Could you check a few things on this model? Use its own coordinates, in mm. A direction names the side the tool comes from. Coordinates: 2 decimals unless noted, no trailing zeros. One line per question, with ' | ' between items. Start each with the question number.
(1) Which directions (+Z, -Z, +X, -X, +Y, -Y) give clear straight access to the entire face, cutting with the end or side of a thin tool? Please do faces 1 (the face through (-72.28, 1.01, -83.14)), 2 (the face through (72.28, 1.01, 83.14)), 3 (the face through (-58.285, 1.014, -97.427)), 4 (the face through (60.1, 1, 85.3)).
(2) Suppose I cut it at A-A (y = 1.15). Give the number of separate pieces and of enclosed holes in the cut face, plus the area to 3 significant figures.
(3) If I drill on line 1 along Z through (x, y) = (-22, 1.9); line 2 along X through (y, z) = (1.2, -13.5); line 3 along X through (y, z) = (0.2, 96), over which ranges is the centre line in solid material (lowest first)?
(4) If we mould it in two halves opening along X, with no side actions, what happens to faces 5 (the face through (-1, 0, -1)), 6 (the face through (72.28, 1.01, -83.14)), 7 (the face through (-58.285, 1.014, 97.427))? For each: pulls with the +X half, pulls with the -X half, needs draft (parallel to the pull), parting line crosses it, or undercut.
```python
from build123d import *

# Parameters (mm, degrees)
SKETCH2_W           = 160
SKETCH2_H           = 210
SKETCH2_R           = 1.3
BOSS_EXTRUDE1_DEPTH = 2
SKETCH3_W           = 14
SKETCH3_H           = 20
CUT_EXTRUDE1_DEPTH  = 2
FILLET1_R           = 1.5
SKETCH4_R           = 1.3
CUT_EXTRUDE2_DEPTH  = 2
CUT_EXTRUDE3_DEPTH  = 2
SKETCH6_R           = 1.65
CUT_EXTRUDE4_DEPTH  = 2


with BuildPart() as part:
    # Sketch2 → Boss-Extrude1 (new body)
    with BuildSketch(Plane(origin=(0, 0, 0), x_dir=(1, 0, 0), z_dir=(0, 1, 0))):
        Rectangle(SKETCH2_W, SKETCH2_H)
        with Locations(Location((52.422835534, 88.736544033, 0), (0, 0, 270))):
            Circle(SKETCH2_R, mode=Mode.SUBTRACT)
        with Locations(Location((52.422835534, 96.514718626, 0), (0, 0, 270))):
            Circle(SKETCH2_R, mode=Mode.SUBTRACT)
        with Locations(Location((58.079689783, 102.171572875, 0), (0, 0, 270))):
            Circle(SKETCH2_R, mode=Mode.SUBTRACT)
        with Locations(Location((76, 13.5, 0), (0, 0, 270))):
            Circle(SKETCH2_R, mode=Mode.SUBTRACT)
        with Locations(Location((68, 13.5, 0), (0, 0, 270))):
            Circle(SKETCH2_R, mode=Mode.SUBTRACT)
        with Locations(Location((62.5, 8, 0), (0, 0, 270))):
            Circle(SKETCH2_R, mode=Mode.SUBTRACT)
        with Locations(Location((62.5, -8, 0), (0, 0, 90))):
            Circle(SKETCH2_R, mode=Mode.SUBTRACT)
        with Locations(Location((68, -13.5, 0), (0, 0, 90))):
            Circle(SKETCH2_R, mode=Mode.SUBTRACT)
        with Locations(Location((76, -13.5, 0), (0, 0, 90))):
            Circle(SKETCH2_R, mode=Mode.SUBTRACT)
        with Locations(Location((77.171572875, 83.079689783, 0), (0, 0, 90))):
            Circle(SKETCH2_R, mode=Mode.SUBTRACT)
        with Locations(Location((71.514718626, 77.422835534, 0), (0, 0, 90))):
            Circle(SKETCH2_R, mode=Mode.SUBTRACT)
        with Locations(Location((63.736544033, 77.422835534, 0), (0, 0, 90))):
            Circle(SKETCH2_R, mode=Mode.SUBTRACT)
        with Locations(Location((77.171572875, -83.079689783, 0), (0, 0, 270))):
            Circle(SKETCH2_R, mode=Mode.SUBTRACT)
        with Locations(Location((71.514718626, -77.422835534, 0), (0, 0, 270))):
            Circle(SKETCH2_R, mode=Mode.SUBTRACT)
        with Locations(Location((63.736544033, -77.422835534, 0), (0, 0, 270))):
            Circle(SKETCH2_R, mode=Mode.SUBTRACT)
        with Locations(Location((58.079689783, -102.171572875, 0), (0, 0, 90))):
            Circle(SKETCH2_R, mode=Mode.SUBTRACT)
        with Locations(Location((52.422835534, -96.514718626, 0), (0, 0, 90))):
            Circle(SKETCH2_R, mode=Mode.SUBTRACT)
        with Locations(Location((52.422835534, -88.736544033, 0), (0, 0, 90))):
            Circle(SKETCH2_R, mode=Mode.SUBTRACT)
        with Locations(Location((-58.079689783, 102.171572875, 0), (0, 0, 90))):
            Circle(SKETCH2_R, mode=Mode.SUBTRACT)
        with Locations(Location((-52.422835534, 96.514718626, 0), (0, 0, 90))):
            Circle(SKETCH2_R, mode=Mode.SUBTRACT)
        with Locations(Location((-52.422835534, 88.736544033, 0), (0, 0, 90))):
            Circle(SKETCH2_R, mode=Mode.SUBTRACT)
        with Locations(Location((-77.171572875, 83.079689783, 0), (0, 0, 270))):
            Circle(SKETCH2_R, mode=Mode.SUBTRACT)
        with Locations(Location((-71.514718626, 77.422835534, 0), (0, 0, 270))):
            Circle(SKETCH2_R, mode=Mode.SUBTRACT)
        with Locations(Location((-63.736544033, 77.422835534, 0), (0, 0, 270))):
            Circle(SKETCH2_R, mode=Mode.SUBTRACT)
        with Locations(Location((-77.171572875, -83.079689783, 0), (0, 0, 90))):
            Circle(SKETCH2_R, mode=Mode.SUBTRACT)
        with Locations(Location((-71.514718626, -77.422835534, 0), (0, 0, 90))):
            Circle(SKETCH2_R, mode=Mode.SUBTRACT)
        with Locations(Location((-63.736544033, -77.422835534, 0), (0, 0, 90))):
            Circle(SKETCH2_R, mode=Mode.SUBTRACT)
        with Locations(Location((-52.422835534, -88.736544033, 0), (0, 0, 270))):
            Circle(SKETCH2_R, mode=Mode.SUBTRACT)
        with Locations(Location((-52.422835534, -96.514718626, 0), (0, 0, 270))):
            Circle(SKETCH2_R, mode=Mode.SUBTRACT)
        with Locations(Location((-58.079689783, -102.171572875, 0), (0, 0, 270))):
            Circle(SKETCH2_R, mode=Mode.SUBTRACT)
        with Locations(Location((-62.5, -8, 0), (0, 0, 270))):
            Circle(SKETCH2_R, mode=Mode.SUBTRACT)
        with Locations(Location((-68, -13.5, 0), (0, 0, 270))):
            Circle(SKETCH2_R, mode=Mode.SUBTRACT)
        with Locations(Location((-76, -13.5, 0), (0, 0, 270))):
            Circle(SKETCH2_R, mode=Mode.SUBTRACT)
        with Locations(Location((-76, 13.5, 0), (0, 0, 90))):
            Circle(SKETCH2_R, mode=Mode.SUBTRACT)
        with Locations(Location((-68, 13.5, 0), (0, 0, 90))):
            Circle(SKETCH2_R, mode=Mode.SUBTRACT)
        with Locations(Location((-62.5, 8, 0), (0, 0, 90))):
            Circle(SKETCH2_R, mode=Mode.SUBTRACT)
    extrude(amount=BOSS_EXTRUDE1_DEPTH)

    # Sketch3 → Cut-Extrude1 (cut)
    with BuildSketch(Plane(origin=(0, 2, 0), x_dir=(1, 0, 0), z_dir=(0, 1, 0))):
        with Locations((73, 0)):
            Rectangle(SKETCH3_W, SKETCH3_H)
        Polygon((65.857864376, 105), (53.129942315, 92.272077939), (67.272077939, 78.129942315), (80, 90.857864376), (80, 105), align=None)
        Polygon((80, -90.857864376), (80, -105), (65.857864376, -105), (53.129942315, -92.272077939), (67.272077939, -78.129942315), align=None)
        Polygon((-80, 90.857864376), (-80, 105), (-65.857864376, 105), (-53.129942315, 92.272077939), (-67.272077939, 78.129942315), align=None)
        with Locations((-73, 0)):
            Rectangle(SKETCH3_W, SKETCH3_H)
        Polygon((-67.272077939, -78.129942315), (-80, -90.857864376), (-80, -105), (-65.857864376, -105), (-53.129942315, -92.272077939), align=None)
    extrude(amount=-CUT_EXTRUDE1_DEPTH, mode=Mode.SUBTRACT)

    # Fillet1
    fillet1_edges = [part.edges().sort_by_distance(p)[0] for p in [
        (65.857864376, 1, -105),
        (80, 1, -90.857864376),
        (80, 1, 90.857864376),
        (65.857864376, 1, 105),
        (-80, 1, -90.857864376),
        (-65.857864376, 1, -105),
        (-80, 1, 10),
        (-80, 1, -10),
        (-65.857864376, 1, 105),
        (-80, 1, 90.857864376),
        (80, 1, -10),
        (80, 1, 10),
    ]]
    fillet(fillet1_edges, radius=FILLET1_R)

    # Sketch4 → Cut-Extrude2 (cut)
    with BuildSketch(Plane(origin=(0, 2, 0), x_dir=(1, 0, 0), z_dir=(0, 1, 0))):
        with Locations(Location((-39, 81.5, 0), (0, 0, 270))):
            Circle(SKETCH4_R)
        with Locations(Location((19, 81.5, 0), (0, 0, 270))):
            Circle(SKETCH4_R)
        with Locations(Location((19, 32.5, 0), (0, 0, 270))):
            Circle(SKETCH4_R)
        with Locations(Location((-39, 32.5, 0), (0, 0, 270))):
            Circle(SKETCH4_R)
    extrude(amount=-CUT_EXTRUDE2_DEPTH, mode=Mode.SUBTRACT)

    # Sketch5 → Cut-Extrude3 (cut)
    with BuildSketch(Plane(origin=(0, 2, 0), x_dir=(1, 0, 0), z_dir=(0, 1, 0))):
        with BuildLine():
            Line((-48, -56.188660248), (-68, -56.188660248))
            ThreePointArc((-68, -56.188660248), (-69.64999998, -57.838916868), (-67.999486759, -59.488660168))
            Line((-67.999486759, -59.488660168), (-47.856342163, -59.482394541))
            ThreePointArc((-47.856342163, -59.482394541), (-46.351567171, -57.766763041), (-48, -56.188660248))
        make_face()
        with BuildLine():
            Line((-48, -36.188660248), (-68, -36.188660248))
            ThreePointArc((-68, -36.188660248), (-69.64999998, -37.838916868), (-67.999486759, -39.488660168))
            Line((-67.999486759, -39.488660168), (-47.856342163, -39.482394541))
            ThreePointArc((-47.856342163, -39.482394541), (-46.351567171, -37.766763041), (-48, -36.188660248))
        make_face()
        with BuildLine():
            Line((-48, -16.188660248), (-68, -16.188660248))
            ThreePointArc((-68, -16.188660248), (-69.64999998, -17.838916868), (-67.999486759, -19.488660168))
            Line((-67.999486759, -19.488660168), (-47.856342163, -19.482394541))
            ThreePointArc((-47.856342163, -19.482394541), (-46.351567171, -17.766763041), (-48, -16.188660248))
        make_face()
        with BuildLine():
            Line((-28.143657837, -19.482394541), (-8.000513241, -19.488660168))
            ThreePointArc((-8.000513241, -19.488660168), (-6.35000002, -17.838916868), (-8, -16.188660248))
            Line((-8, -16.188660248), (-28, -16.188660248))
            ThreePointArc((-28, -16.188660248), (-29.648432829, -17.766763041), (-28.143657837, -19.482394541))
        make_face()
        with BuildLine():
            Line((-28.143657837, -39.482394541), (-8.000513241, -39.488660168))
            ThreePointArc((-8.000513241, -39.488660168), (-6.35000002, -37.838916868), (-8, -36.188660248))
            Line((-8, -36.188660248), (-28, -36.188660248))
            ThreePointArc((-28, -36.188660248), (-29.648432829, -37.766763041), (-28.143657837, -39.482394541))
        make_face()
        with BuildLine():
            Line((-28.143657837, -59.482394541), (-8.000513241, -59.488660168))
            ThreePointArc((-8.000513241, -59.488660168), (-6.35000002, -57.838916868), (-8, -56.188660248))
            Line((-8, -56.188660248), (-28, -56.188660248))
            ThreePointArc((-28, -56.188660248), (-29.648432829, -57.766763041), (-28.143657837, -59.482394541))
        make_face()
    extrude(amount=-CUT_EXTRUDE3_DEPTH, mode=Mode.SUBTRACT)

    # Sketch6 → Cut-Extrude4 (cut)
    with BuildSketch(Plane(origin=(0, 2, 0), x_dir=(1, 0, 0), z_dir=(0, 1, 0))):
        with Locations(Location((8.790094163, -66.528420774, 0), (0, 0, 270))):
            Circle(SKETCH6_R)
        with Locations(Location((8.790094163, -12.828420774, 0), (0, 0, 270))):
            Circle(SKETCH6_R)
        with Locations(Location((53.490094163, -12.828420774, 0), (0, 0, 270))):
            Circle(SKETCH6_R)
        with Locations(Location((53.490094163, -66.528420774, 0), (0, 0, 270))):
            Circle(SKETCH6_R)
    extrude(amount=-CUT_EXTRUDE4_DEPTH, mode=Mode.SUBTRACT)


solid = part.part
```
Checks:
1) face 1: -Z, +Y, -Y | face 2: +Z, +Y, -Y | face 3: -X, +Y, -Y | face 4: +Y, -Y
2) separate pieces: 1 | enclosed holes: 50 | area: 30,500 mm^2
3) line 1: z = -105 to 16.19, 19.48 to 36.19, 39.48 to 56.19, 59.48 to 105 | line 2: x = -80 to -77.3, -74.7 to -69.3, -66.7 to 66.7, 69.3 to 74.7, 77.3 to 80 | line 3: x = -56.86 to -53.62, -51.23 to 51.23, 53.62 to 56.86
4) face 5: needs draft | face 6: undercut | face 7: pulls with the -X half
